Part model, mm, in its own coordinate system. A direction names the side the tool comes from. Give positions to 0.01 mm unless a question says otherwise; leave off trailing zeros. Order: outer loops, then holes, each group sorted by start corner. A loop starts at its lowest first (then second) coordinate and runs counter-clockwise, first axis right, second up. Notation, with made-up numbers: M 77.25,-30 L 100.25,-30 A17 cw 100.25,-4 Z; hole C 68,61 d1. An arc over 180 degrees is marked long. Answer as a JSON object with one key per item and string values.
from build123d import *

# Parameters (mm, degrees)
SKETCH1_W           = 34
SKETCH1_H           = 70
SKETCH1_W_2         = 22
SKETCH1_H_2         = 42
BOSS_EXTRUDE1_DEPTH = 3
CUT_EXTRUDE1_DEPTH  = 44.874821937
CHAMFER1_SIZE       = 2
SKETCH3_W           = 7
SKETCH3_H           = 7
CUT_EXTRUDE2_DEPTH  = 3
SKETCH4_W           = 24
SKETCH4_H           = 50
SKETCH4_R           = 2
BOSS_EXTRUDE2_DEPTH = 2
CHAMFER2_SIZE       = 2
BOSS_EXTRUDE3_START = -10
BOSS_EXTRUDE3_DEPTH = 2
BOSS_EXTRUDE4_START = -40
BOSS_EXTRUDE4_DEPTH = 2
FILLET1_R           = 0.5


with BuildPart() as part:
    # Sketch1 → Boss-Extrude1 (new, symmetric)
    with BuildSketch(Plane(origin=(0, 0, 0), x_dir=(0, 0, -1), z_dir=(1, 0, 0))):
        with Locations((0, -5)):
            Rectangle(SKETCH1_W, SKETCH1_H)
        Rectangle(SKETCH1_W_2, SKETCH1_H_2, mode=Mode.SUBTRACT)
    extrude(amount=BOSS_EXTRUDE1_DEPTH, both=True)

    # Sketch2 → Cut-Extrude1 (cut, through all)
    with BuildSketch(Plane.ZY.offset(3)):
        with BuildLine():
            Line((-6.5, -21), (-6.5, -22))
            ThreePointArc((-6.5, -22), (-5, -26.5), (-3.5, -22))
            Line((-3.5, -22), (-3.5, -21))
            Line((-3.5, -21), (-6.5, -21))
        make_face()
        with BuildLine():
            Line((3.5, -21), (3.5, -22))
            ThreePointArc((3.5, -22), (5, -26.5), (6.5, -22))
            Line((6.5, -22), (6.5, -21))
            Line((6.5, -21), (3.5, -21))
        make_face()
        with BuildLine():
            Line((6.5, 21), (6.5, 22))
            ThreePointArc((6.5, 22), (5, 26.5), (3.5, 22))
            Line((3.5, 22), (3.5, 21))
            Line((3.5, 21), (6.5, 21))
        make_face()
        with BuildLine():
            Line((-3.5, 21), (-3.5, 22))
            ThreePointArc((-3.5, 22), (-5, 26.5), (-6.5, 22))
            Line((-6.5, 22), (-6.5, 21))
            Line((-6.5, 21), (-3.5, 21))
        make_face()
    extrude(amount=-CUT_EXTRUDE1_DEPTH, mode=Mode.SUBTRACT)

    # Chamfer1
    chamfer1_edges = [part.edges().sort_by_distance(p)[0] for p in [
        (3, -5, 17),
        (3, 30, 0),
        (-3, -5, 17),
        (-3, -5, -17),
        (-3, 30, 0),
        (3, -5, -17),
        (0, 30, 17),
        (0, 30, -17),
    ]]
    chamfer(chamfer1_edges, length=CHAMFER1_SIZE)

    # Sketch3 → Cut-Extrude2 (cut)
    with BuildSketch(Plane(origin=(3, 0, 0), x_dir=(0, 0, -1), z_dir=(1, 0, 0))):
        with Locations((5, 24)):
            Rectangle(SKETCH3_W, SKETCH3_H)
        with Locations((5, -24)):
            Rectangle(SKETCH3_W, SKETCH3_H)
        with Locations((-5, -24)):
            Rectangle(SKETCH3_W, SKETCH3_H)
        with Locations((-5, 24)):
            Rectangle(SKETCH3_W, SKETCH3_H)
    extrude(amount=-CUT_EXTRUDE2_DEPTH, mode=Mode.SUBTRACT)

    # Sketch4 → Boss-Extrude2 (add)
    with BuildSketch(Plane.XZ.offset(40)):
        with Locations((9, 0)):
            Rectangle(SKETCH4_W, SKETCH4_H)
        with Locations(Location((1, -21, 0), (0, 0, 270))):
            Circle(SKETCH4_R, mode=Mode.SUBTRACT)
        with Locations(Location((17, -21, 0), (0, 0, 270))):
            Circle(SKETCH4_R, mode=Mode.SUBTRACT)
        with Locations(Location((17, 21, 0), (0, 0, 270))):
            Circle(SKETCH4_R, mode=Mode.SUBTRACT)
        with Locations(Location((1, 21, 0), (0, 0, 270))):
            Circle(SKETCH4_R, mode=Mode.SUBTRACT)
    extrude(amount=-BOSS_EXTRUDE2_DEPTH)

    # Chamfer2
    chamfer2_edges = [part.edges().sort_by_distance(p)[0] for p in [
        (-3, -39, -25),
        (-3, -39, 25),
        (21, -39, 25),
        (21, -39, -25),
    ]]
    chamfer(chamfer2_edges, length=CHAMFER2_SIZE)

    # Sketch5 → Boss-Extrude3 (add)
    with BuildSketch(Plane(origin=(0, 0, -25), x_dir=(-1, 0, 0), z_dir=(0, 0, -1)).offset(BOSS_EXTRUDE3_START)):
        Polygon((-3, -38), (-21, -38), (-3, -5), align=None)
    extrude(amount=-BOSS_EXTRUDE3_DEPTH)

    # Sketch5<2> → Boss-Extrude4 (add)
    with BuildSketch(Plane(origin=(0, 0, -25), x_dir=(-1, 0, 0), z_dir=(0, 0, -1)).offset(BOSS_EXTRUDE4_START)):
        Polygon((-3, -38), (-21, -38), (-3, -5), align=None)
    extrude(amount=BOSS_EXTRUDE4_DEPTH)

    # Fillet1
    fillet1_edges = [part.edges().sort_by_distance(p)[0] for p in [
        (3, 21, -9.75),
        (3, 24.25, -8.5),
        (3, 27.5, -5),
        (3, 24.25, -1.5),
        (3, -21, -9.75),
        (3, -24.25, -1.5),
        (3, -27.5, -5),
        (3, -24.25, -8.5),
        (3, 21, 9.75),
        (3, 0, 11),
        (3, -21, 9.75),
        (3, -21, 0),
        (3, 0, -11),
        (3, -24.25, 8.5),
        (3, -27.5, 5),
        (3, -24.25, 1.5),
        (3, 21, 0),
        (3, 24.25, 1.5),
        (3, 27.5, 5),
        (3, 24.25, 8.5),
        (12, -21.5, -13),
        (12, -21.5, -15),
        (12, -21.5, 13),
        (12, -21.5, 15),
    ]]
    fillet(fillet1_edges, radius=FILLET1_R - 0.0001)  # a hair under: the kernel refuses the full size


solid = part.part
1. Cut at A-A on z = -21. Give the cut face in (x, y), plus the area to 3 significant figures.
Worked answers:
{"outline": "M -3,-40 L -1,-40 L -1,-38 L -3,-38 Z; M 3,-40 L 15,-40 L 15,-38 L 3,-38 Z; M 19,-40 L 21,-40 L 21,-38 L 19,-38 Z", "area": "32.0 mm^2"}
2. Which spindle directions (+Z, -Z, +X, -X, +Y, -Y) get a long thin tool onto all of the face, cutting with end or side? Do faces 5 (the flat face through (2, -5, 16)), 6 (the flat face through (-2, -5, -16)), 7 (the flat face through (12, -38, 0)). Say none if no direction does.
Worked answers:
{"face 5": "+Z, +X, +Y", "face 6": "-Z, -X, +Y", "face 7": "+X, +Y"}
3. Cut at D-D on y = -3.5. Give the cut face in (x, z), plus the area to 3 significant figures.
Worked answers:
{"outline": "M -3,-15 L -1,-17 L 1,-17 L 3,-15 L 3,-11.5 A0.5 ccw 2.5,-11 L -3,-11 Z; M -3,11 L 2.5,11 A0.5 ccw 3,11.5 L 3,15 L 1,17 L -1,17 L -3,15 Z", "area": "63.9 mm^2"}
4. Two-plate mould, pull along Y, no slides. Class faces 1 (the flat face through (0, 26, -3)), 2 (the flat face through (0, 0, -11)), 3 (the cylindrical face through (-0.2, -39, 22.6)), 4 (the flat face through (1.6, 28.8, 15.6)): +Y half, -Y half, draft (parallel to the pull), parting line (faces both ways), or undercut.
Worked answers:
{"face 1": "undercut", "face 2": "undercut", "face 3": "draft", "face 4": "+Y half"}
5. Pin check, flat tips, straight feed: P1, Ø14, axis at x = 9.5, y = -24, coming from the -Z side; P2, Ø3, axis at y = -25.5, z = -4.5, coming from the +X side; P3, Ø14, axis at x = 11.5, y = -15.5, coming from the +Z side. Stop position of each tip, or through.
Worked answers:
{"P1": "stops at z = -15.5", "P2": "stops at x = 0", "P3": "stops at z = 15"}
6. Cut at B-B on y = 24. Give the cut face in (x, z).
Worked answers:
{"outline": "M -3,-15 L -1,-17 L 1,-17 L 3,-15 L 3,-9 A0.5 ccw 2.5,-8.5 L 0,-8.5 L 0,-7.5 L -3,-7.5 Z; M -3,-2.5 L 0,-2.5 L 0,-1.5 L 2.5,-1.5 A0.5 ccw 3,-1 L 3,1 A0.5 ccw 2.5,1.5 L 0,1.5 L 0,2.5 L -3,2.5 Z; M -3,7.5 L 0,7.5 L 0,8.5 L 2.5,8.5 A0.5 ccw 3,9 L 3,15 L 1,17 L -1,17 L -3,15 Z"}
7. Probe line 1 along Z through (x, y) = (12.25, -36); line 2 along Y through (x, z) = (2.5, 17); line 3 along Y through (x, z) = (-0.9, 5). List the from-to ranges inside material, lowest first.
Worked answers:
{"line 1": "z = -15 to -13, 13 to 15", "line 2": "y = -40 to -38", "line 3": "y = -40 to -26.5, 26.5 to 30"}
